Drawing for the job (mm, zero at the part's lowest x, y, z). A direction names the side the tool comes from. Give positions to 0.01 mm unless a question says otherwise; leave off trailing zeros. Order: outer loops, then holes, each group sorted by start corner. A loop starts at its lowest first (then second) coordinate and runs counter-clockwise, first axis right, second up. Notation, with made-up numbers: (16, 46) - (59, 46) arc R34 cw to (59, 84) - close; hole circle Ø7 at (21, 45). An arc over 180 degrees is marked (long way). Use a Markdown table: item, result.
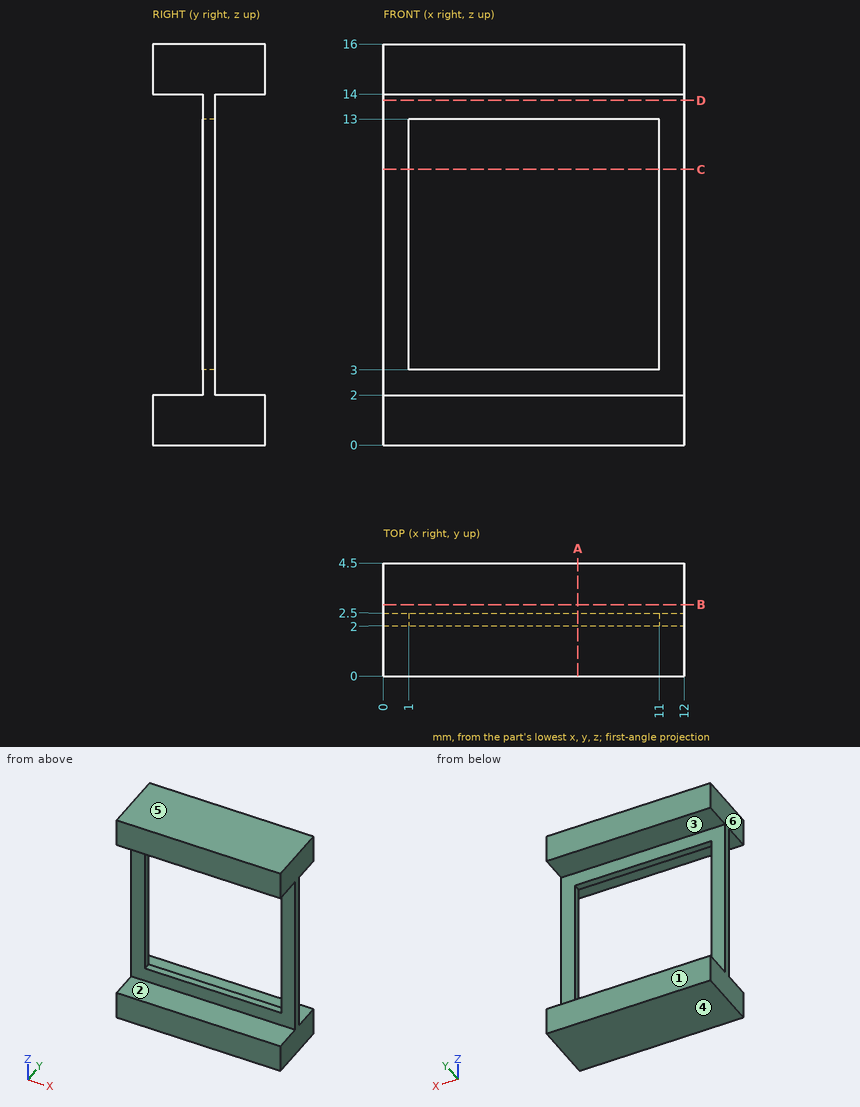
1) Tool access for the marked faces 1 and 2: list every direction of +Z, -Z, +X, -X, +Y, -Y with a clear straight run to the whole face (end or side of a thin tool).
Computed:
| item | result |
|---|---|
| face 1 | +Z, -Z, +X, -X, +Y |
| face 2 | +X, -X, -Y |
2) Slice it at D-D (z = 13.75). Write the cut outline in (x, y), and give its area (3 significant figures).
Computed:
| item | result |
|---|---|
| outline | (0, 2) - (12, 2) - (12, 2.5) - (0, 2.5) - close |
| area | 6.00 mm² |
3) Pin check, flat tip, straight feed: P1, Ø3.5, axis at x = 3, z = 6.5, coming from the +Y side. Stop position of the tip, or through.
Computed:
| item | result |
|---|---|
| P1 | passes through |
4) Slice it at A-A (x = 7.75). Write the cut outline in (y, z), and give its area (3 significant figures).
Computed:
| item | result |
|---|---|
| outline | (0, 0) - (4.5, 0) - (4.5, 2) - (2.5, 2) - (2.5, 3) - (2, 3) - (2, 2) - (0, 2) - close; (0, 14) - (2, 14) - (2, 13) - (2.5, 13) - (2.5, 14) - (4.5, 14) - (4.5, 16) - (0, 16) - close |
| area | 19.0 mm² |
5) Wall check: line 1 (Z direction, x = 10.5, y = 1.95); line 2 (Z direction, x = 4, y = 2.3); line 3 (Y direction, x = 1.5, z = 2.75). Give the ranges that are in metal, low to high. Write a range as from..to.
Computed:
| item | result |
|---|---|
| line 1 | z = 0..2, 14..16 |
| line 2 | z = 0..3, 13..16 |
| line 3 | y = 2..2.5 |
6) Two-plate mould, pull along Z, no slides. Class the marked faces 3, 4, 5 and 6: +Z half, -Z half, draft (parallel to the pull), parting line (faces both ways), or undercut.
Computed:
| item | result |
|---|---|
| face 3 | undercut |
| face 4 | -Z half |
| face 5 | +Z half |
| face 6 | draft |
7) Slice it at B-B (y = 2.85). Write the cut outline in (x, z).
Computed:
| item | result |
|---|---|
| outline | (0, 0) - (12, 0) - (12, 2) - (0, 2) - close; (0, 14) - (12, 14) - (12, 16) - (0, 16) - close |
8) Slice it at C-C (z = 11). Write the cut outline in (x, y).
Computed:
| item | result |
|---|---|
| outline | (0, 2) - (1, 2) - (1, 2.5) - (0, 2.5) - close; (11, 2) - (12, 2) - (12, 2.5) - (11, 2.5) - close |
